Read the model definition and answer for the solid it produces. Units are mm, in the model's axes. A direction names the side the tool comes from. Coordinates: 2 decimals unless noted, no trailing zeros. Loops run counter-clockwise (first coordinate to the right, second up) from the corner with the lowest first, then second, coordinate; pieces in that order, holes last.
from build123d import *

# Parameters (mm, degrees)
SKETCH_1_W                   = 81
SKETCH_1_H                   = 30
EXTRUDE_1_DEPTH              = 10
HOLE_WIZARD_M5_1_D           = 5.8
HOLE_WIZARD_M5_1_CBORE_D     = 10
HOLE_WIZARD_M5_1_CBORE_DEPTH = 5
SKETCH_4_W                   = 81
SKETCH_4_H                   = 12
CUT_EXTRUDE_1_DEPTH          = 2
CUT_EXTRUDE_2_DEPTH          = 85.273364713
CUT_EXTRUDE_2_DEPTH_BACK     = 85.273364713
SKETCH_5_W                   = 34
SKETCH_5_H                   = 2
HOLE_WIZARD_M4_1_D           = 3.3


with BuildPart() as part:
    # 草图1 → 凸台-拉伸1 (new body)
    with BuildSketch(Plane.XY):
        with Locations((40.5, 15)):
            Rectangle(SKETCH_1_W, SKETCH_1_H)
    extrude(amount=EXTRUDE_1_DEPTH)

    # M5 六角凹头螺钉的柱形沉头孔1 (through all)
    with Locations(Plane(origin=(0, 0, 0), x_dir=(-1, 0, 0), z_dir=(0, 0, -1))):
        with Locations((-34, 15), (-8, 15)):
            CounterBoreHole(HOLE_WIZARD_M5_1_D / 2, HOLE_WIZARD_M5_1_CBORE_D / 2, HOLE_WIZARD_M5_1_CBORE_DEPTH)

    # 草图4 → 切除-拉伸1 (cut)
    with BuildSketch(Plane.XY.offset(10)):
        with Locations((40.5, 15)):
            Rectangle(SKETCH_4_W, SKETCH_4_H)
    extrude(amount=-CUT_EXTRUDE_1_DEPTH, mode=Mode.SUBTRACT)

    # 草图5 → 切除-拉伸2 (cut, two sides: drawn at the far end of the back side and taken through both)
    with BuildSketch(Plane.XZ.offset(-21).offset(-CUT_EXTRUDE_2_DEPTH_BACK)):
        with Locations((64, 9)):
            Rectangle(SKETCH_5_W, SKETCH_5_H)
    extrude(amount=CUT_EXTRUDE_2_DEPTH + CUT_EXTRUDE_2_DEPTH_BACK, mode=Mode.SUBTRACT)

    # M4 螺纹孔1 (through all)
    with Locations(Plane.XY.offset(8)):
        with Locations((71.3, 15), (61.3, 15)):
            Hole(HOLE_WIZARD_M4_1_D / 2)


solid = part.part
Item 1: Which of the six approach directions +Z, -Z, +X, -X, +Y, -Y give full straight-line access (tool end or side, diameter ignored) to faces 4 (the face through (47, 5, 9)), 5 (the face through (23, 9, 9)), 6 (the face through (72.95, 15.07, 3.94)), 7 (the face through (31.8, 12.8, 5))?
Numbers:
face 4: +Z, +X, +Y, -Y
face 5: +Z, +X, -X
face 6: +Z, -Z
face 7: -Z
Item 2: A cutting plane is placed at D-D on y = 19. Determine the outline of the cut face in (x, z), then the cut area to 3 significant figures.
Numbers:
outline: (0, 0) - (5, 0) - (5, 5) - (11, 5) - (11, 0) - (31, 0) - (31, 5) - (37, 5) - (37, 0) - (81, 0) - (81, 8) - (0, 8) - close
area: 588 mm2
Item 3: Determine the mould class of faces 1 (the face through (81, 15, 4)), 2 (the face through (23, 5, 10)), 3 (the face through (5.693, 10.564, 2.465)) for opening direction X: released by +X, released by -X, zero draft, split by the parting line, or undercut.
Numbers:
face 1: released by +X
face 2: zero draft
face 3: undercut
Item 4: A cutting plane is placed at C-C on x = 38. Determine the outline of the cut face in (y, z).
Numbers:
outline: (0, 0) - (12, 0) - (12, 5) - (18, 5) - (18, 0) - (30, 0) - (30, 10) - (21, 10) - (21, 8) - (9, 8) - (9, 10) - (0, 10) - close
Item 5: Given pin 1 (1.5 mm diameter, centred on x = 38, y = 14.5, fed in from +Z); pin 2 (0.6 mm diameter, centred on y = 5, z = 8.5, fed in from +X); pin 3 (1 mm diameter, centred on x = 32.5, y = 11.5, fed in from -Z), each flat-ended and moving along its own axis, determine where each tip first touches the part or whether it passes through.
Numbers:
pin 1: stops at z = 8
pin 2: stops at x = 47
pin 3: stops at z = 5
Item 6: A cutting plane is placed at A-A on y = 15. Determine the outline of the cut face in (x, z).
Numbers:
outline: (0, 0) - (3, 0) - (3, 5) - (5.1, 5) - (5.1, 8) - (0, 8) - close; (10.9, 5) - (13, 5) - (13, 0) - (29, 0) - (29, 5) - (31.1, 5) - (31.1, 8) - (10.9, 8) - close; (36.9, 5) - (39, 5) - (39, 0) - (59.65, 0) - (59.65, 8) - (36.9, 8) - close; (62.95, 0) - (69.65, 0) - (69.65, 8) - (62.95, 8) - close; (72.95, 0) - (81, 0) - (81, 8) - (72.95, 8) - close
Item 7: Find the intervals of material crossed by line 1 along Y through (x, z) = (24, 9); line 2 along X through (y, z) = (16.5, 4.25); line 3 along Z through (x, y) = (7, 20.25), in increasing order.
Numbers:
line 1: y = 0 to 9, 21 to 30
line 2: x = 0 to 3.23, 12.77 to 29.23, 38.77 to 60.61, 61.99 to 70.61, 71.99 to 81
line 3: z = 0 to 8
Item 8: A cutting plane is placed at B-B on x = 8. Determine the outline of the cut face in (y, z).
Numbers:
outline: (0, 0) - (10, 0) - (10, 5) - (12.1, 5) - (12.1, 8) - (9, 8) - (9, 10) - (0, 10) - close; (17.9, 5) - (20, 5) - (20, 0) - (30, 0) - (30, 10) - (21, 10) - (21, 8) - (17.9, 8) - close
